```python
from build123d import *

# Parameters (mm, degrees)
SKETCH_1_R      = 2.5
EXTRUDE_1_DEPTH = 3


with BuildPart() as part:
    # 草图1 → 凸台-拉伸1 (new body)
    with BuildSketch(Plane(origin=(0, 0, 0), x_dir=(1, 0, 0), z_dir=(0, 1, 0))):
        with BuildLine():
            ThreePointArc((0, 2), (0.585786438, 0.585786438), (2, 0))
            Line((2, 0), (33, 0))
            ThreePointArc((33, 0), (34.414213562, -0.585786438), (35, -2))
            Line((35, -2), (35, -43))
            ThreePointArc((35, -43), (35.585786438, -44.414213562), (37, -45))
            Line((37, -45), (48, -45))
            ThreePointArc((48, -45), (49.414213562, -44.414213562), (50, -43))
            Line((50, -43), (50, 0))
            Line((50, 0), (50, 18))
            ThreePointArc((50, 18), (49.414213562, 19.414213562), (48, 20))
            Line((48, 20), (2, 20))
            ThreePointArc((2, 20), (0.585786438, 19.414213562), (0, 18))
            Line((0, 18), (0, 2))
        make_face()
        with Locations(Location((42.5, -32.5, 0), (0, 0, 270))):
            Circle(SKETCH_1_R, mode=Mode.SUBTRACT)
        with Locations(Location((10, 10, 0), (0, 0, 270))):
            Circle(SKETCH_1_R, mode=Mode.SUBTRACT)
        with Locations(Location((25, 10, 0), (0, 0, 270))):
            Circle(SKETCH_1_R, mode=Mode.SUBTRACT)
        with Locations(Location((42.5, 7.5, 0), (0, 0, 270))):
            Circle(SKETCH_1_R, mode=Mode.SUBTRACT)
    extrude(amount=EXTRUDE_1_DEPTH)


solid = part.part
```
Geometry: final body of the model. Coordinates: model frame, mm. A direction names the side the tool comes from. Round coordinates to 2 decimals unless told otherwise and drop trailing zeros. Write each loop counter-clockwise with the first axis right and the second up, starting at its lowest first coordinate (ties: lowest second). Pieces come first, ordered by that corner, then holes.
Item 1: Section query A-A (x = 10). Return loops of the section in (y, z), plus the area to 3 significant figures.
Item 2: Material intervals for L1, parallel to X at y = 2.3, z = 32.5; L2, parallel to X at y = 1, z = 11; L3, parallel to Z at x = 10.5, y = 1, sorted ascending.
Item 3: Section query B-B (y = 0.6). Return loops of the section in (x, z).
Item 4: Set-up query: faces 4 (the face through (42, 1, 45)), 5 (the face through (35, 1, 22)). Return all of +Z, -Z, +X, -X, +Y, -Y with unobstructed straight access to the full face (end or side cutting, diameter ignored); none if empty.
Item 5: Mould query, pull axis Z, two halves, no side actions, for faces 1 (the face through (49.43, 1.48, -19.4)), 2 (the face through (27.48, 1.48, -10.33)), 3 (the face through (49.4, 1.48, 44.43)). Classes: +Z half, -Z half, draft (parallel to the pull), parting line (faces both ways), or undercut.
Item 6: Section query C-C (z = 32.5). Return loops of the section in (x, y).
Item 7: Section query D-D (x = 42.5). Return loops of the section in (y, z).
Item 8: Pin query (flat end, axial travel): P1, Ø6.5, axis at x = 42.5, z = -7.5, coming from the -Y side; P2, Ø1.5, axis at x = 7, y = 1, coming from the +Z side. Return the tip coordinate at first contact, or that it passes through.
Completed:
1. outline: (0, -20) - (3, -20) - (3, -12.5) - (0, -12.5) - close; (0, -7.5) - (3, -7.5) - (3, 0) - (0, 0) - close
1. area: 45.0 mm2
2. L1: x = 35 to 40, 45 to 50
2. L2: x = 35 to 50
2. L3: z = -20 to -12.45, -7.55 to 0
3. outline: (0, -18) arc R2 ccw to (2, -20) - (48, -20) arc R2 ccw to (50, -18) - (50, 43) arc R2 ccw to (48, 45) - (37, 45) arc R2 ccw to (35, 43) - (35, 2) arc R2 cw to (33, 0) - (2, 0) arc R2 ccw to (0, -2) - close; hole circle Ø5 at (10, -10); hole circle Ø5 at (25, -10); hole circle Ø5 at (42.5, -7.5); hole circle Ø5 at (42.5, 32.5)
4. face 4: +Z, +X, -X, +Y, -Y
4. face 5: +Z, -X, +Y, -Y
5. face 1: -Z half
5. face 2: undercut
5. face 3: +Z half
6. outline: (35, 0) - (40, 0) - (40, 3) - (35, 3) - close; (45, 0) - (50, 0) - (50, 3) - (45, 3) - close
7. outline: (0, -20) - (3, -20) - (3, -10) - (0, -10) - close; (0, -5) - (3, -5) - (3, 30) - (0, 30) - close; (0, 35) - (3, 35) - (3, 45) - (0, 45) - close
8. P1: stops at y = 0
8. P2: stops at z = 0
